The listing builds one solid part. Answer for the finished solid, in the listing's coordinates (mm). A direction names the side the tool comes from. Coordinates: 2 decimals unless noted, no trailing zeros. Write each loop counter-clockwise with the first axis right and the second up, starting at its lowest first coordinate (ties: lowest second). Pieces come first, ordered by that corner, then holes. Notation, with made-up numbers: M 12,-30 L 45,-30 A18 cw 45,-13 Z; hole C 64.5,61 d2. An arc over 180 degrees is marked long. Answer as a JSON object with one key per item and string values. Group by question number.
Autodesk Inventor part; units mm, degrees
ref_plane "YZ Plane" through (0, 0, 0) normal (1, 0, 0) x (0, 1, 0)
ref_plane "XZ Plane" through (0, 0, 0) normal (0, 1, 0) x (-1, 0, 0)
ref_plane "XY Plane" through (0, 0, 0) normal (0, 0, 1) x (1, 0, 0)
sketch "Sketch2" plane through (0, 0, 0) normal (0, 0, 1) x (1, 0, 0)
  line L0 (-25.5, 40) -> (25.5, 40)
  line L1 (25.5, 40) -> (25.5, -40)
  line L2 (25.5, -40) -> (-25.5, -40)
  line L3 (-25.5, -40) -> (-25.5, 40)
  line L4 (-25.5, 40) -> (25.5, -40) construction
  line L5 (25.5, 40) -> (-25.5, -40) construction
  line L6 (-25.5, 0) -> (-10.25, 0) construction
  line L7 (25.5, 0) -> (10.25, 0) construction
  line L8 (-10.25, -25) -> (-10.25, 25) construction
  line L9 (-7.5, -25) -> (-7.5, 25)
  line L10 (-13, 25) -> (-13, -25)
  arc A0 (-13, -25) -> (-7.5, -25) centre (-10.25, -25) ccw
  arc A1 (-7.5, 25) -> (-13, 25) centre (-10.25, 25) ccw
  line L11 (10.25, -25) -> (10.25, 25) construction
  line L12 (13, -25) -> (13, 25)
  line L13 (7.5, 25) -> (7.5, -25)
  arc A2 (7.5, -25) -> (13, -25) centre (10.25, -25) ccw
  arc A3 (13, 25) -> (7.5, 25) centre (10.25, 25) ccw
  point P0 (0, 0)
  dimension "d2" = 51
  dimension "d3" = 80
  dimension "d4" = 15.25
  dimension "d5" = 15.25
  dimension "d6" = 25
  dimension "d7" = 5.5
  dimension "d8" = 25
  dimension "d9" = 5.5
extrude "Extrusion1" add sketch "Sketch2" along normal blind 3
sketch "Sketch3" plane through (0, 0, 3) normal (0, 0, 1) x (1, 0, 0)
  line L0 (25.5, -40) -> (25.5, 40)
  line L1 (-25.5, -40) -> (25.5, -40)
  line L2 (25.5, -40) -> (25.5, -37)
  line L3 (25.5, -37) -> (-25.5, -37)
  line L4 (-25.5, -37) -> (-25.5, -40)
  point P0 (0, 0)
  dimension "d12" = 3
extrude "Extrusion2" add sketch "Sketch3" along normal blind 35
sketch "Sketch4" plane through (-25.5, -37, 3) normal (0, 1, 0) x (1, 0, 0)
  line L0 (0, 0) -> (51, 0) construction
  line L1 (25.5, 0) -> (25.5, -35) construction
  line L2 (51, -35) -> (0, -35) construction
  line L3 (0, 3) -> (0, -35) construction
  line L4 (0, -17.5) -> (15.25, -17.5) construction
  line L5 (0, -17.5) -> (15.25, -17.5) construction
  line L6 (51, 0) -> (51, -35) construction
  line L7 (51, -17.5) -> (35.75, -17.5) construction
  line L8 (15.25, -23.5) -> (15.25, -11.5) construction
  line L9 (18, -23.5) -> (18, -11.5)
  line L10 (12.5, -11.5) -> (12.5, -23.5)
  arc A0 (12.5, -23.5) -> (18, -23.5) centre (15.25, -23.5) ccw
  arc A1 (18, -11.5) -> (12.5, -11.5) centre (15.25, -11.5) ccw
  line L11 (35.75, -23.5) -> (35.75, -11.5) construction
  line L12 (38.5, -23.5) -> (38.5, -11.5)
  line L13 (33, -11.5) -> (33, -23.5)
  arc A2 (33, -23.5) -> (38.5, -23.5) centre (35.75, -23.5) ccw
  arc A3 (38.5, -11.5) -> (33, -11.5) centre (35.75, -11.5) ccw
  point P0 (25.5, 3)
  dimension "d15" = 15.25
  dimension "d17" = 15.25
  dimension "d18" = 6
  dimension "d19" = 5.5
  dimension "d20" = 6
  dimension "d21" = 5.5
extrude "Extrusion3" cut sketch "Sketch4" against normal through all
fillet "Fillet2" radius 25 2 edges at (-25.5, -38.5, 38) (25.5, -38.5, 38)
properties part number "Vertical_L_Bracket" material "Aluminum 6061"
Item 1: A cutting plane is placed at B-B, the plane z = 16. Write down the section's boundary in (x, y).
Item 2: A cutting plane is placed at C-C, the plane x = -10.25. Write down the section's boundary in (y, z).
Item 3: A cutting plane is placed at A-A, the plane y = -15.5. Write down the section's boundary in (x, z).
Item 4: A tool of negligible diameter and unlimited length cuts with its end or side. For faces 1 (the face through (13, -38, 21)), 2 (the face through (10.19, 27.75, 1.48)), 3 (the face through (17.982, -38.479, 30.871)), from which of +Z, -Z, +X, -X, +Y, -Y can it reach the whole face along a straight path? Write none if from no direction.
Item 5: Consider L1, parallel to Y at x = 10, z = 2; L2, parallel to Z at x = 4.5, y = -23; L3, parallel to Y at x = 11.5, z = 34.5. Determine where each line is inside the solid, lowest interval first. Write a range as from..to.
Item 6: Flat-ended cylindrical pins translate along their axes: pin 1 Ø1.5 at (x, z) = (18.5, 29.5) entering from +Y; pin 2 Ø3.5 at (y, z) = (-39, 17.5) entering from +X; pin 3 Ø2 at (x, y) = (-19, -4) entering from +Z. Find the tip coordinate at first contact, or state that the pin passes through.
Item 7: A cutting plane is placed at D-D, the plane x = -18. Write down the section's boundary in (y, z), and give its area (3 significant figures).
Item 8: For a pull along Y with two mould halves and no side action, classify faces 4 (the face through (-10.19, -38.48, 11.75)), 5 (the face through (0, -40, 15)), 6 (the face through (10.31, -27.75, 1.48)) as +Y half, -Y half, draft (parallel to the pull), parting line (faces both ways), or undercut.
Answer:
{
 "1": {"outline": "M -25.32,-40 L -13,-40 L -13,-37 L -25.32,-37 Z; M -7.5,-40 L 7.5,-40 L 7.5,-37 L -7.5,-37 Z; M 13,-40 L 25.32,-40 L 25.32,-37 L 13,-37 Z"},
 "2": {"outline": "M -40,0 L -27.75,0 L -27.75,3 L -37,3 L -37,11.75 L -40,11.75 Z; M -40,29.25 L -37,29.25 L -37,36.02 L -40,36.02 Z; M 27.75,0 L 40,0 L 40,3 L 27.75,3 Z"},
 "3": {"outline": "M -25.5,0 L -13,0 L -13,3 L -25.5,3 Z; M -7.5,0 L 7.5,0 L 7.5,3 L -7.5,3 Z; M 13,0 L 25.5,0 L 25.5,3 L 13,3 Z"},
 "4": {"face 1": "+Y, -Y", "face 2": "+Z, -Z", "face 3": "+Z, +X, +Y, -Y"},
 "5": {"L1": "-40..-27.74, 27.74..40", "L2": "0..3", "L3": "-40..-37"},
 "6": {"pin 1": "y = -37", "pin 2": "x = 25.35", "pin 3": "z = 3"},
 "7": {"outline": "M -40,0 L 40,0 L 40,3 L -37,3 L -37,30.85 L -40,30.85 Z", "area": "324 mm2"},
 "8": {"face 4": "draft", "face 5": "-Y half", "face 6": "undercut"}
}
